Read the model definition and answer for the solid it produces. Units are mm, in the model's axes. A direction names the side the tool comes from. Coordinates: 2 decimals unless noted, no trailing zeros. Write each loop counter-clockwise with the first axis right and the second up, starting at its lowest first coordinate (ties: lowest second). Pieces come first, ordered by that corner, then holes. Notation, with made-up numbers: (41, 41) -> (94, 41) arc R16 cw to (94, 61) -> close; hole circle Ø7 at (28.5, -33). An arc over 180 degrees is marked (long way). Answer as a JSON object with one key per item and string values. Group by question number.
(1) Straight lines are drawn through the part: L1, parallel to Y at x = 27.5, z = 1.3 (3 decimals); L2, parallel to X at y = -4.5, z = 2.75; L3, parallel to X at y = 16.5, z = 0.95 (1 decimal). For each, find the intervals that lie inside material, in ascending order.
(2) Flat-ended cylindrical pins translate along their axes: P1, Ø5.5, axis at x = -19.5, y = 3.5, coming from the -Z side; P2, Ø13, axis at x = -15.5, y = 0, coming from the -Z side. Find the tip coordinate at first contact, or state that the pin passes through.
(3) Find section B-B (y = -3.5). Give the vertices of the cut face in (x, z).
(4) For a pull along Y with two mould halves and no side action, classify faces 3 (the face through (-26.75, 0, 3)), 4 (the face through (28.21, 16.72, 4.99)), 5 (the face through (-16.953, -14.109, 3.324)), 6 (the face through (-28.93, -17.4, 2.03)) as +Y half, -Y half, draft (parallel to the pull), parting line (faces both ways), or undercut.
(5) Find section C-C (x = 12.5). Give the vertices of the cut face in (y, z), then the cut area to 3 significant figures.
(6) Find section A-A (x = 22). Give the vertices of the cut face in (y, z).
(7) Which of the six approach directions +Z, -Z, +X, -X, +Y, -Y give full straight-line access (tool end or side, diameter ignored) to faces 1 (the face through (-28.5, -0.2, 5)), 2 (the face through (26, 15.25, 3))?
from build123d import *
from OCP.BRepFilletAPI import BRepFilletAPI_MakeChamfer

# Parameters (mm, degrees)
SKETCH_1_W          = 59
SKETCH_1_H          = 36
EXTRUDE_1_DEPTH     = 6
SKETCH_2_W          = 53.5
SKETCH_2_H          = 30.5
CUT_EXTRUDE_1_DEPTH = 5.2
FILLET_1_R          = 2
SKETCH_3_W          = 4
SKETCH_3_H          = 30.5
EXTRUDE_2_DEPTH     = 3.7
FILLET_2_R          = 4
CHAMFER_1_SIZE      = 2
SKETCH_4_W          = 11
SKETCH_4_H          = 5.2
CUT_EXTRUDE_2_DEPTH = 10
FILLET_3_R          = 0.2
CHAMFER_2_SIZE      = 0.2
CHAMFER_2_SIZE_2    = 0.141421356
M1_2X0_25_1_D       = 0.95
M1_2X0_25_1_DEPTH   = 3
M1_2X0_25_1_TIP     = 0.285408794


with BuildPart() as part:
    # 草图1 → 凸台-拉伸1 (new body)
    with BuildSketch(Plane.XY):
        Rectangle(SKETCH_1_W, SKETCH_1_H)
    extrude(amount=EXTRUDE_1_DEPTH)

    # 草图2 → 切除-拉伸1 (cut)
    with BuildSketch(Plane(origin=(0, 0, 0), x_dir=(-1, 0, 0), z_dir=(0, 0, -1))):
        Rectangle(SKETCH_2_W, SKETCH_2_H)
    extrude(amount=-CUT_EXTRUDE_1_DEPTH, mode=Mode.SUBTRACT)

    # 圆角1
    fillet_1_edges = [part.edges().sort_by_distance(p)[0] for p in [
        (29.5, -18, 3),
        (-29.5, -18, 3),
        (-29.5, 18, 3),
        (29.5, 18, 3),
    ]]
    fillet(fillet_1_edges, radius=FILLET_1_R)

    # 草图3 → 凸台-拉伸2 (add)
    with BuildSketch(Plane(origin=(0, 0, 5.2), x_dir=(-1, 0, 0), z_dir=(0, 0, -1))):
        with Locations((13.75, 0)):
            Rectangle(SKETCH_3_W, SKETCH_3_H)
    extrude(amount=EXTRUDE_2_DEPTH)

    # 圆角2
    fillet_2_edges = [part.edges().sort_by_distance(p)[0] for p in [
        (-15.75, -15.25, 3.35),
        (-15.75, 15.25, 3.35),
        (-11.75, 15.25, 3.35),
        (-11.75, -15.25, 3.35),
    ]]
    fillet(fillet_2_edges, radius=FILLET_2_R)

    # 倒角1
    chamfer_1_edges = [part.edges().sort_by_distance(p)[0] for p in [
        (-29.5, 0, 6),
        (0, 18, 6),
        (29.5, 0, 6),
        (0, -18, 6),
        (28.914213562, -17.414213562, 6),
        (28.914213562, 17.414213562, 6),
        (-28.914213562, -17.414213562, 6),
        (-28.914213562, 17.414213562, 6),
    ]]
    chamfer(chamfer_1_edges, length=CHAMFER_1_SIZE)

    # 草图4 → 切除-拉伸2 (cut)
    with BuildSketch(Plane(origin=(0, 18, 0), x_dir=(1, 0, 0), z_dir=(0, 1, 0))):
        with Locations((20, -2.6)):
            Rectangle(SKETCH_4_W, SKETCH_4_H)
    extrude(amount=-CUT_EXTRUDE_2_DEPTH, mode=Mode.SUBTRACT)

    # 圆角3
    fillet_3_edges = [part.edges().sort_by_distance(p)[0] for p in [
        (-26.75, 15.25, 2.6),
        (-26.75, -15.25, 2.6),
        (26.75, -15.25, 2.6),
        (26.75, 15.25, 2.6),
    ]]
    fillet(fillet_3_edges, radius=FILLET_3_R)

    # 倒角2
    chamfer_2_edges_1 = [part.edges().sort_by_distance(p)[0] for p in [
        (14.5, 17.4, 4.6),
        (25.5, 17.4, 4.6),
        (25.5, 18, 2),
        (14.5, 18, 2),
    ]]
    chamfer_2_edges_2 = [part.edges().sort_by_distance(p)[0] for p in [
        (20, 16.8, 5.2),
    ]]
    chamfer_2_side_2 = [part.faces().sort_by_distance(p)[0] for p in [
        (20, 16.797171573, 5.2),
    ]]
    chamfer_2 = BRepFilletAPI_MakeChamfer(part.part.solid().wrapped)
    for e in chamfer_2_edges_1:
        chamfer_2.Add(CHAMFER_2_SIZE - 0.0001, e.wrapped)
    for e in chamfer_2_edges_2:
        chamfer_2.Add(CHAMFER_2_SIZE_2 - 0.0001, CHAMFER_2_SIZE - 0.0001, e.wrapped, chamfer_2_side_2[0].wrapped)
    add(Compound.cast(chamfer_2.Shape()), mode=Mode.REPLACE)  # a hair under: the kernel refuses the full size

    # M1.2x0.25 螺纹孔1
    with Locations(Plane(origin=(27.5, 16.5, 0), x_dir=(-1, 0, 0), z_dir=(0, 0, -1))):
        with Locations((0, 0), (0, -33), (55, -33), (55, 0)):
            Hole(M1_2X0_25_1_D / 2, depth=M1_2X0_25_1_DEPTH)
            with Locations((0, 0, -(M1_2X0_25_1_DEPTH + M1_2X0_25_1_TIP / 2))):  # 118° drill point
                Cone(0, M1_2X0_25_1_D / 2, M1_2X0_25_1_TIP, mode=Mode.SUBTRACT)


solid = part.part
Results below:
{
 "1": {"L1": "y = -18 to -16.975, -16.025 to 16.025, 16.975 to 18", "L2": "x = -29.5 to -26.75, -15.75 to -11.75, 26.75 to 29.5", "L3": "x = -29.4 to -28, -27 to 14.5, 25.5 to 27, 28 to 29.4"},
 "2": {"P1": "stops at z = 5.2", "P2": "stops at z = 1.5"},
 "3": {"outline": "(-29.5, 0) -> (-26.75, 0) -> (-26.75, 5.2) -> (-15.75, 5.2) -> (-15.75, 1.5) -> (-11.75, 1.5) -> (-11.75, 5.2) -> (26.75, 5.2) -> (26.75, 0) -> (29.5, 0) -> (29.5, 4) -> (27.5, 6) -> (-27.5, 6) -> (-29.5, 4) -> close"},
 "4": {"face 3": "undercut", "face 4": "+Y half", "face 5": "undercut", "face 6": "-Y half"},
 "5": {"outline": "(-18, 0) -> (-15.25, 0) -> (-15.25, 5.2) -> (15.25, 5.2) -> (15.25, 0) -> (18, 0) -> (18, 4) -> (16, 6) -> (-16, 6) -> (-18, 4) -> close", "area": "53.4 mm2"},
 "6": {"outline": "(-18, 0) -> (-15.25, 0) -> (-15.25, 5.2) -> (16.66, 5.2) -> (16.66, 5.34) -> (16, 6) -> (-16, 6) -> (-18, 4) -> close"},
 "7": {"face 1": "+Z, -X, +Y, -Y", "face 2": "-Z"}
}
